Can you work these out from the model? Positions are in its coordinate system, mm. A direction names the side the tool comes from. Coordinates: 2 decimals unless noted, no trailing zeros. Order: outer loops, then holes, each group sorted by start corner. A loop starts at its lowest first (then second) coordinate and runs counter-clockwise, first axis right, second up. Notation, with made-up numbers: (-1, 40.5) -> (3, 40.5) arc R7 ccw to (3, 46.5) -> close; hole circle Ø4 at (-14.5, 13.25). An arc over 180 degrees is marked (long way). Use a Markdown table: item, result. Add a question column.
1. Suppose I cut it at A-A, the plane y = -0.25. List the corners of the cut face in (x, z) for me.
2. Suppose I cut it at C-C, the plane z = 6.75. List the corners of the cut face in (x, y) for me.
3. For pin 1 Ø1 at (x, z) = (1, 6.5) entering from -Y, with a flat end and sliding along its axis, tell me the tip position at first contact or that it passes through.
4. Suppose I cut it at B-B, the plane x = 4.1. List the corners of the cut face in (y, z) for me.
5. If I drill on line 1 along Y through (x, z) = (3.5, 1.25); line 2 along X through (y, z) = (3, 1), over which ranges is the centre line in solid material (lowest first)? Write a range as from..to.
6. For faces 1 (the flat face through (0, 6.56, 7)), 2 (the cylindrical face through (-3.832, -0.611, 0.985)), which set-ups out of +Z, -Z, +X, -X, +Y, -Y let a thin tool reach every point of the face, with its end or its side?
```python
from build123d import *

# Parameters (mm, degrees)
CYLINDER006_R     = 0.58
CYLINDER006_DEPTH = 1.24
BOX013_W          = 11.52
BOX013_H          = 6.56
BOX013_DEPTH      = 13.2
FILLET011_R       = 1.5
CYLINDER007_R     = 0.58
CYLINDER007_DEPTH = 1.24


with BuildPart() as cylinder006:
    # Cylinder006 → Cylinder006 (new body)
    with BuildSketch(Plane(origin=(-4.1, 0, 1.5), x_dir=(1, 0, 0), z_dir=(0, -1, 0))):
        Circle(CYLINDER006_R)
    extrude(amount=CYLINDER006_DEPTH)


with BuildPart() as fusion002:
    # Box013 → Box013 (new body)
    with BuildSketch(Plane(origin=(-5.76, 0, 0), x_dir=(1, 0, 0), z_dir=(0, 0, 1))):
        with Locations((5.76, 3.28)):
            Rectangle(BOX013_W, BOX013_H)
    extrude(amount=BOX013_DEPTH)

    # Fillet011
    fillet011_edges = [fusion002.edges().sort_by_distance(p)[0] for p in [
        (-5.76, 3.28, 13.2),
        (-5.76, 3.28, 0),
        (5.76, 3.28, 13.2),
        (5.76, 3.28, 0),
    ]]
    fillet(fillet011_edges, radius=FILLET011_R)

    # Fusion002: union Cylinder006
    add(cylinder006.part)


with BuildPart() as encoderbody:
    # Cylinder007 → Cylinder007 (new body)
    with BuildSketch(Plane(origin=(4.1, 0, 11.7), x_dir=(1, 0, 0), z_dir=(0, -1, 0))):
        Circle(CYLINDER007_R)
    extrude(amount=CYLINDER007_DEPTH)

    # Fusion003: union Fusion002
    add(fusion002.part)


solid = encoderbody.part
```
Worked out:
| question | item | result |
|---|---|---|
| 1 | outline | circle Ø1.16 at (-4.1, 1.5); circle Ø1.16 at (4.1, 11.7) |
| 2 | outline | (-5.76, 0) -> (5.76, 0) -> (5.76, 6.56) -> (-5.76, 6.56) -> close |
| 3 | pin 1 | stops at y = 0 |
| 4 | outline | (-1.24, 11.12) -> (0, 11.12) -> (0, 0) -> (6.56, 0) -> (6.56, 13.2) -> (0, 13.2) -> (0, 12.28) -> (-1.24, 12.28) -> close |
| 5 | line 1 | y = 0..6.56 |
| 5 | line 2 | x = -5.67..5.67 |
| 6 | face 1 | +Z, -Z, +X, -X, +Y |
| 6 | face 2 | -Y |
